Answer from the drawing. Dimensions are ordinates in mm from the lowest x, y and z of the part. A direction names the side the tool comes from. Give positions to 0.01 mm unless a question says otherwise; leave off trailing zeros. Loops run counter-clockwise (first coordinate to the right, second up) from the corner with the lowest first, then second, coordinate; pieces in that order, holes last.
(1) Each of these flat-tipped pins is pushed along its axis until it touches: P1, Ø4, axis at x = 3, y = 1.5, coming from the -Z side; P2, Ø1.5, axis at y = 8.5, z = 5, coming from the -X side. Where does it stop, or does it pass through?
(2) Find section D-D, the plane x = 1. Write down the section's boundary in (y, z).
(3) Find section B-B, the plane x = 3.25. Write down the section's boundary in (y, z), then the cut area to 3 significant figures.
(4) Straight lines are drawn through the part: probe 1 along Y at (x, z) = (5.75, 4.5); probe 2 along Y at (x, z) = (0.5, 4). For each, find the intervals that lie inside material, in ascending order.
(5) Find section C-C, the plane y = 13.5. Write down the section's boundary in (x, z).
(6) Find section A-A, the plane z = 4.5. Write down the section's boundary in (x, y).
(7) Which of the six approach directions +Z, -Z, +X, -X, +Y, -Y give full straight-line access (tool end or side, diameter ignored) to the marked faces 1, 2, 3 and 4?
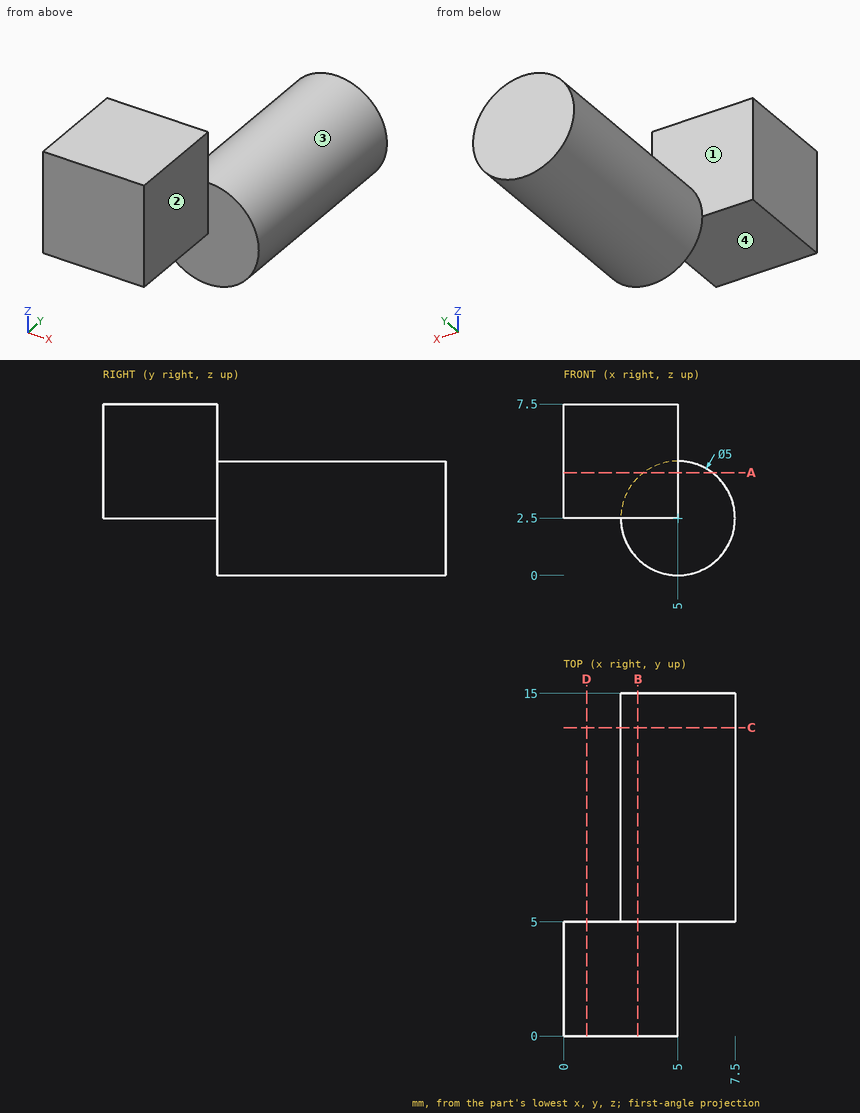
Entries:
1. P1: stops at z = 2.5
1. P2: stops at x = 3.21
2. outline: (0, 2.5) - (5, 2.5) - (5, 7.5) - (0, 7.5) - close
3. outline: (0, 2.5) - (5, 2.5) - (5, 0.71) - (15, 0.71) - (15, 4.29) - (5, 4.29) - (5, 7.5) - (0, 7.5) - close
3. area: 60.7 mm2
4. probe 1: y = 5 to 15
4. probe 2: y = 0 to 5
5. outline: circle Ø5 at (5, 2.5)
6. outline: (0, 0) - (5, 0) - (5, 5) - (6.5, 5) - (6.5, 15) - (3.5, 15) - (3.5, 5) - (0, 5) - close
7. face 1: +Z, -X, +Y
7. face 2: +Z, -Z, +X, -Y
7. face 3: +Y
7. face 4: -Z, +X, -X, -Y
